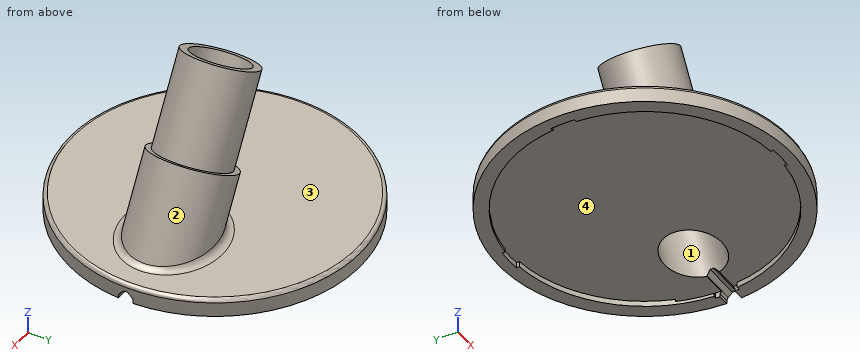
Autodesk Fusion 360 part; units mm, degrees
sketch "Skizze1" plane through (0, 0, 0) normal (0, 0, 1) x (1, 0, 0)
  circle A0 centre (0, 0) radius 80
extrude "Extrusion1" add sketch "Skizze1" along normal blind 10 makes body 1
fillet "Abrundung1" radius 2 1 edges at (-74.5862, -28.9292, 10) on bodies 1
sketch "Skizze2" plane through (0, 0, 0) normal (0, 1, 0) x (1, 0, 0)
  line L0 (45, 0) -> (-5, -86.6025) construction
ref_plane "Arbeitsebene1" through (-5, 0, 86.6025) normal (-0.5, 0, 0.866) x (0, -1, 0)
sketch "Skizze3" plane through (-5, 0, 86.6025) normal (-0.5, 0, 0.866) x (0, -1, 0)
  circle A0 centre (0, 0) radius 23
  circle A1 centre (0, 0) radius 20
extrude "Extrusion5" add sketch "Skizze3" against normal blind 110 separate body contours A0 | A1 makes body 2
combine "Kombinieren1" operation add target body 1 tool bodies 2
extrude "Extrusion6" cut sketch "Skizze3" against normal blind 50 bodies 1
fillet "Abrundung2" radius 4 3 edges at (65.7846, 0, 10) (-74.5862, -28.9292, 8) (-72.7215, 28.206, 10) on bodies 1
sketch "Skizze4" plane through (-5, 0, 86.6025) normal (-0.5, 0, 0.866) x (0, -1, 0)
  circle A0 centre (0, 0) radius 15.75
extrude "Extrusion7" cut sketch "Skizze4" against normal blind 110 bodies 1
sketch "Skizze5" plane through (0, 0, 0) normal (0, 0, 1) x (1, 0, 0)
  circle A0 centre (0, 0) radius 160
extrude "Extrusion8" cut sketch "Skizze5" against normal blind 110 bodies 1
sketch "Skizze6" plane through (0, 0, 0) normal (0, 0, 1) x (1, 0, 0)
  line L0 (45, 0) -> (85, 0)
ref_plane "Arbeitsebene2" through (45, 0, 0) normal (1, 0, 0) x (0, 1, 0)
sketch "Skizze7" plane through (45, 0, 0) normal (1, 0, 0) x (0, 1, 0)
  line L0 (-4, 0) -> (-4, 1.7)
  line L1 (-4, 1.7) -> (-3.2, 3.3)
  line L2 (-3.2, 3.3) -> (-1, 5.5)
  line L3 (-1, 5.5) -> (1, 5.5)
  line L4 (1, 5.5) -> (3.2, 3.3)
  line L5 (3.2, 3.3) -> (4, 1.7)
  line L6 (4, 1.7) -> (4, 0)
  line L7 (4, 0) -> (-4, 0)
sweep "Sweeping1" cut profiles "Skizze7" path "Skizze6" along L0 section 1 bodies 1
sketch "Skizze8" plane through (0, 0, 0) normal (0, 0, 1) x (1, 0, 0)
  circle A0 centre (0, 0) radius 72.5
extrude "Extrusion9" cut sketch "Skizze8" along normal blind 3 bodies 1
sketch "Skizze9" plane through (0, 0, 0) normal (0, 0, 1) x (1, 0, 0)
  line L0 (72.2241, -6.3188) -> (73.7184, -6.4495)
  arc A0 (73.7184, -6.4495) -> (73.7184, 6.4495) centre (0, 0) ccw
  line L1 (73.7184, 6.4495) -> (72.2241, 6.3188)
  arc A1 (72.2241, -6.3188) -> (72.2241, 6.3188) centre (0, 0) ccw
  line L2 (6.3188, 72.2241) -> (6.4495, 73.7184)
  arc A2 (6.4495, 73.7184) -> (-6.4495, 73.7184) centre (0, 0) ccw
  line L3 (-6.4495, 73.7184) -> (-6.3188, 72.2241)
  arc A3 (6.3188, 72.2241) -> (-6.3188, 72.2241) centre (0, 0) ccw
  line L4 (-72.2241, 6.3188) -> (-73.7184, 6.4495)
  arc A4 (-73.7184, 6.4495) -> (-73.7184, -6.4495) centre (0, 0) ccw
  line L5 (-73.7184, -6.4495) -> (-72.2241, -6.3188)
  arc A5 (-72.2241, 6.3188) -> (-72.2241, -6.3188) centre (0, 0) ccw
  line L6 (-6.3188, -72.2241) -> (-6.4495, -73.7184)
  arc A6 (-6.4495, -73.7184) -> (6.4495, -73.7184) centre (0, 0) ccw
  line L7 (6.4495, -73.7184) -> (6.3188, -72.2241)
  arc A7 (-6.3188, -72.2241) -> (6.3188, -72.2241) centre (0, 0) ccw
extrude "Extrusion10" cut sketch "Skizze9" along normal blind 3 bodies 1
sketch "Skizze10" plane through (0, 0, 0) normal (0, 0, 1) x (1, 0, 0)
  line L0 (72.2241, -6.3188) -> (73.7184, -6.4495)
  arc A0 (73.7184, -6.4495) -> (69.5373, 25.3095) centre (0, 0) ccw
  line L1 (69.5373, 25.3095) -> (68.1277, 24.7965)
  arc A1 (72.2241, -6.3188) -> (68.1277, 24.7965) centre (0, 0) ccw
  line L2 (6.3188, 72.2241) -> (6.4495, 73.7184)
  arc A2 (6.4495, 73.7184) -> (-25.3095, 69.5373) centre (0, 0) ccw
  line L3 (-25.3095, 69.5373) -> (-24.7965, 68.1277)
  arc A3 (6.3188, 72.2241) -> (-24.7965, 68.1277) centre (0, 0) ccw
  line L4 (-72.2241, 6.3188) -> (-73.7184, 6.4495)
  arc A4 (-73.7184, 6.4495) -> (-69.5373, -25.3095) centre (0, 0) ccw
  line L5 (-69.5373, -25.3095) -> (-68.1277, -24.7965)
  arc A5 (-72.2241, 6.3188) -> (-68.1277, -24.7965) centre (0, 0) ccw
  line L6 (-6.3188, -72.2241) -> (-6.4495, -73.7184)
  arc A6 (-6.4495, -73.7184) -> (25.3095, -69.5373) centre (0, 0) ccw
  line L7 (25.3095, -69.5373) -> (24.7965, -68.1277)
  arc A7 (-6.3188, -72.2241) -> (24.7965, -68.1277) centre (0, 0) ccw
extrude "Extrusion11" cut sketch "Skizze10" along normal blind 1.25 from surface at 1.75 bodies 1
sketch "Skizze11" plane through (0, 0, 0) normal (0, 0, 1) x (1, 0, 0)
  circle A0 centre (0, 0) radius 72.2
extrude "Extrusion12" add sketch "Skizze11" along normal blind 3 separate body makes body 3
fillet "Abrundung3" radius 0.5 1 edges at (-67.314, -26.1086, 3) on bodies 3
sketch "Skizze12" plane through (0, 0, 0) normal (0, 0, 1) x (1, 0, 0)
  line L0 (71.0266, -4.9667) -> (73.5205, -5.1411)
  arc A0 (73.5205, -5.1411) -> (73.5205, 5.1411) centre (0, 0) ccw
  line L1 (73.5205, 5.1411) -> (71.0266, 4.9667)
  arc A1 (71.0266, -4.9667) -> (71.0266, 4.9667) centre (0, 0) ccw
  line L2 (4.9667, 71.0266) -> (5.1411, 73.5205)
  arc A2 (5.1411, 73.5205) -> (-5.1411, 73.5205) centre (0, 0) ccw
  line L3 (-5.1411, 73.5205) -> (-4.9667, 71.0266)
  arc A3 (4.9667, 71.0266) -> (-4.9667, 71.0266) centre (0, 0) ccw
  line L4 (-71.0266, 4.9667) -> (-73.5205, 5.1411)
  arc A4 (-73.5205, 5.1411) -> (-73.5205, -5.1411) centre (0, 0) ccw
  line L5 (-73.5205, -5.1411) -> (-71.0266, -4.9667)
  arc A5 (-71.0266, 4.9667) -> (-71.0266, -4.9667) centre (0, 0) ccw
  line L6 (-4.9667, -71.0266) -> (-5.1411, -73.5205)
  arc A6 (-5.1411, -73.5205) -> (5.1411, -73.5205) centre (0, 0) ccw
  line L7 (5.1411, -73.5205) -> (4.9667, -71.0266)
  arc A7 (-4.9667, -71.0266) -> (4.9667, -71.0266) centre (0, 0) ccw
extrude "Extrusion13" add sketch "Skizze12" along normal blind 1.1 from surface at 1.9 separate body makes body 4 at (72.7424, 3.9409, 1.9) makes body 5 at (-72.7424, 3.9409, 1.9) makes body 6 at (-3.9409, 72.7424, 1.9) makes body 7 at (0.5522, -72.8469, 1.9)
combine "Kombinieren2" operation add target body 3 tool bodies 4 5 6 7
sketch "Skizze13" plane through (0, 0, 0) normal (0, 0, 1) x (1, 0, 0)
  circle A0 centre (0, 39.875) radius 9
  circle A1 centre (0, -39.875) radius 9
extrude "Extrusion14" cut sketch "Skizze13" along normal blind 3 bodies 3
delete_body "Körper entfernen1" bodies 3
equation "base_plate_diameter = 160 mm"
equation "base_plate_height = 10 mm"
equation "base_plate_rounding = 2 mm"
equation "leg_outer_diameter = 46 mm"
equation "ring_inner_diameter = 40 mm"
equation "ring_extrude_depth = 50 mm"
equation "hole_inner_diameter = 31.5 mm"
equation "leg_length = 100 mm"
equation "leg_angle = 120 deg"
equation "leg_offset = 45 mm"
equation "leg_plate_rounding = 4 mm"
equation "cable_channel_width = 8 mm"
equation "cable_channel_depth = 5.5 mm"
equation "cable_channel_vertical_height = 2.5 mm"
equation "cable_channel_edge_chamfer = 0.8 mm"
equation "cover_plate_diameter = 145 mm"
equation "cover_plate_thickness = 3 mm"
equation "finger_grip_diameter = 18 mm"
equation "finger_grip_depth = 1.5 mm"
equation "clamp_recess_width = 22 mm"
equation "clamp_recess_length = 12 mm"
equation "clamp_recess_depth = 2.5 mm"
equation "strain_relief_screw_diameter = 2.6 mm"
equation "strain_relief_screw_depth = 6 mm"
equation "d25 = base_plate_height"
equation "d28 = base_plate_rounding"
equation "d41 = leg_plate_rounding"
equation "d53 = cover_plate_thickness"
equation "d55 = cover_plate_thickness"
equation "d60 = cover_plate_thickness"
equation "d67 = cover_plate_thickness"
Could you check a few things on this model? Use its own coordinates, in mm. Face numbers are marked on the shaded views. Coordinates: 2 decimals unless noted, no trailing zeros. Use one line per item in the form item = value. Start each with the question number.
1. Please list where these lines run through material, in increasing order: line 1 (X direction, y = -8, z = 14); line 2 (Z direction, x = -5, y = 3); line 3 (Z direction, x = -24, y = -53).
2. For pin 1 (10 mm diameter, centred on y = 16, z = 60.5, fed in from +X); pin 2 (5 mm diameter, centred on x = 0, z = 36, fed in from +Y); pin 3 (1.6 mm diameter, centred on x = 74, y = -0.5, fed in from -Z), each with a flat end and sliding along its axis, tell me the tip position at first contact or that it passes through.
3. We'd pull the mould along X, two halves only. Please class the marked faces 1, 2, 3 and 4: +X half, -X half, draft (parallel to the pull), parting line (faces both ways), or undercut.
Geometry says:
q1.line_1 = 11.44 to 21.25, 52.58 to 61.82
q1.line_2 = 3 to 10, 47.06 to 55.68
q1.line_3 = 3 to 10
q2.pin_1 = 30.28
q2.pin_2 = 7.67
q2.pin_3 = 5.2
q3.face_1 = undercut
q3.face_2 = parting line
q3.face_3 = draft
q3.face_4 = undercut
